Read the model definition and answer for the solid it produces. Units are mm, in the model's axes. A direction names the side the tool comes from. Coordinates: 2 decimals unless noted, no trailing zeros. Write each loop counter-clockwise with the first axis right and the second up, starting at its lowest first coordinate (ties: lowest second). Pieces come first, ordered by that corner, then holes. Notation, with made-up numbers: (72.25, -20.5) -> (102.25, -20.5) arc R27 cw to (102.25, 7.5) -> close; hole circle Ø8 at (69, -3.75). An arc over 180 degrees is marked (long way). Use CSV: the item, a comma, the result in double quotes. Start each with the question number.
from build123d import *

# Parameters (mm, degrees)
SKETCH_1_R          = 3
EXTRUDE_1_DEPTH     = 22
SKETCH_1_3_R        = 5
SKETCH_1_3_R_2      = 3
EXTRUDE_2_DEPTH     = 3
SKETCH_2_W          = 1.5
SKETCH_2_H          = 10
CUT_EXTRUDE_1_DEPTH = 1.5


with BuildPart() as part:
    # Sketch 1 → Extrude 1 (new body)
    with BuildSketch(Plane.XY):
        Circle(SKETCH_1_R)
    extrude(amount=EXTRUDE_1_DEPTH)

    # Sketch 1_3 → Extrude 2 (add)
    with BuildSketch(Plane.XY):
        Circle(SKETCH_1_3_R)
        Circle(SKETCH_1_3_R_2, mode=Mode.SUBTRACT)
        Circle(SKETCH_1_3_R_2)
    extrude(amount=-EXTRUDE_2_DEPTH)

    # Sketch 2 → Cut-Extrude 1 (cut)
    with BuildSketch(Plane(origin=(0, 0, -3), x_dir=(-1, 0, 0), z_dir=(0, 0, -1))):
        Rectangle(SKETCH_2_W, SKETCH_2_H)
    extrude(amount=-CUT_EXTRUDE_1_DEPTH, mode=Mode.SUBTRACT)


solid = part.part
1) Find the intervals of material crossed by line 1 along Z through (x, y) = (0, 2.5); line 2 along Z through (x, y) = (3, 1); line 3 along X through (y, z) = (-1.5, 11.5), in increasing order.
2) Section C-C, the plane z = 15 is taken. Give the vertices of the cut face in (x, y).
3) Which of the six approach directions +Z, -Z, +X, -X, +Y, -Y give full straight-line access (tool end or side, diameter ignored) to faces 4 (the face through (-0.1, -3.3, 0)), 5 (the face through (-0.75, 0, -2)), 6 (the face through (0, 0, 22))?
4) Each of these flat-tipped pins is pushed along its axis until it touches: pin 1 (5 mm diameter, centred on x = -2.5, z = 9, fed in from +Y); pin 2 (3 mm diameter, centred on x = -3.5, y = -4, fed in from +Z); pin 3 (1.5 mm diameter, centred on x = -3, z = 1.5, fed in from -Y). Where does it stop, or does it pass through?
5) The mould has two halves that part along X. Classify faces 1 (the face through (-1.08, -4.88, -1.48)), 2 (the face through (0, 0, -1.5)), 3 (the face through (2, 0, -3)): pulls with the +X half, pulls with the -X half, needs draft (parallel to the pull), parting line crosses it, or undercut.
6) Section B-B, the plane y = 0 is taken. Give the vertices of the cut face in (x, z), plus the area to 3 significant figures.
7) Section D-D, the plane y = 3.75 is taken. Give the vertices of the cut face in (x, z).
8) Section A-A, the plane x = 0 is taken. Give the vertices of the cut face in (y, z), plus the area to 3 significant figures.
The answers:
1,line 1,"z = -1.5 to 22"
1,line 2,"z = -3 to 0"
1,line 3,"x = -2.6 to 2.6"
2,outline,"circle Ø6 at (0, 0)"
3,face 4,"+Z"
3,face 5,"-Z, +Y, -Y"
3,face 6,"+Z, +X, -X, +Y, -Y"
4,pin 1,"stops at y = 3"
4,pin 2,"stops at z = 0"
4,pin 3,"stops at y = -1.98"
5,face 1,"parting line crosses it"
5,face 2,"undercut"
5,face 3,"needs draft"
6,outline,"(-5, -3) -> (-0.75, -3) -> (-0.75, -1.5) -> (0.75, -1.5) -> (0.75, -3) -> (5, -3) -> (5, 0) -> (3, 0) -> (3, 22) -> (-3, 22) -> (-3, 0) -> (-5, 0) -> close"
6,area,"160 mm^2"
7,outline,"(-3.31, -3) -> (-0.75, -3) -> (-0.75, -1.5) -> (0.75, -1.5) -> (0.75, -3) -> (3.31, -3) -> (3.31, 0) -> (-3.31, 0) -> close"
8,outline,"(-5, -1.5) -> (5, -1.5) -> (5, 0) -> (3, 0) -> (3, 22) -> (-3, 22) -> (-3, 0) -> (-5, 0) -> close"
8,area,"147 mm^2"
